Source: CAD feature listing. Evaluate the final solid. Frame: model axes, mm. Face numbers are marked on the shaded views. Give positions to 0.01 mm unless a question says otherwise; leave off trailing zeros. Loops run counter-clockwise (first coordinate to the right, second up) from the corner with the lowest first, then second, coordinate; pieces in that order, holes last. Notation, with made-up numbers: (29, 29.5) -> (87, 29.5) arc R24 cw to (87, 68.5) -> close; hole circle Ø7 at (43.5, 59). An arc over 180 degrees is marked (long way). Put each result on its own line as item: value.
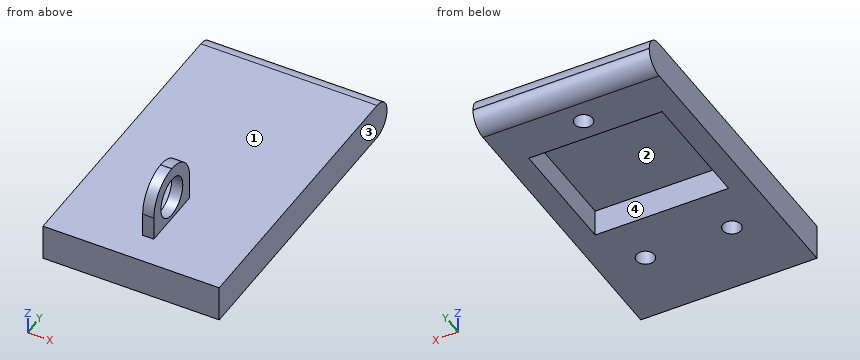
```python
from build123d import *

# Parameters (mm, degrees)
F0_W     = 3.1
F0_H     = 18.1
F1_DEPTH = 25.75
F0_W_2   = 48.9
F0_H_2   = 84.6
F2_DEPTH = 10.1
F3_R     = 5
F4_R     = 9
F5_R     = 5.499402
F6_DEPTH = 26.001
F7_R     = 2.5
F7_W     = 37
F7_H     = 33.5
F8_DEPTH = 7.5


with BuildPart() as f1:
    # F0 (on Top) → F1 (new body)
    with BuildSketch(Plane.XY):
        with Locations((23.972543, 18.115168)):
            Rectangle(F0_W, F0_H)
    extrude(amount=F1_DEPTH)

    # F0 (on Top) → F2 (join)
    with BuildSketch(Plane.XY):
        with Locations((23.972543, 42.723387)):
            Rectangle(F0_W_2, F0_H_2)
        with Locations((23.972543, 18.115168)):
            Rectangle(F0_W, F0_H, mode=Mode.SUBTRACT)
    extrude(amount=F2_DEPTH)

    # F3
    f3_edges = [f1.edges().sort_by_distance(p)[0] for p in [
        (23.972543, 85.023387, 10.1),
        (23.972543, 85.023387, 0),
    ]]
    fillet(f3_edges, radius=F3_R)

    # F4
    f4_edges = [f1.edges().sort_by_distance(p)[0] for p in [
        (23.972543, 9.065168, 25.75),
        (23.972543, 27.165168, 25.75),
    ]]
    fillet(f4_edges, radius=F4_R)

    # F5 (on face) → F6 (cut, through all)
    with BuildSketch(Plane.YZ.offset(25.522543)):
        with Locations((18.165168, 16.75)):
            Circle(F5_R)
    extrude(amount=-F6_DEPTH, mode=Mode.SUBTRACT)

    # F7 (on face) → F8 (cut)
    with BuildSketch(Plane.XY):
        with Locations((23.972543, 73.70657)):
            Circle(F7_R)
        with Locations((35.972543, 20.70657)):
            Circle(F7_R)
        with Locations((11.972543, 20.70657)):
            Circle(F7_R)
        with Locations((23.972543, 50.95657)):
            Rectangle(F7_W, F7_H)
    extrude(amount=F8_DEPTH, mode=Mode.SUBTRACT)


solid = f1.part
```
(1) Line query: probe 1 along X at (y, z) = (64, 1.5); probe 2 along X at (y, z) = (18.5, 5); probe 3 along X at (y, z) = (22, 11.5). Output: solid intervals per line, ascending. Write a range as from..to.
Calculated:
probe 1: x = -0.48..5.47, 42.47..48.42
probe 2: x = -0.48..10.8, 13.15..34.8, 37.15..48.42
probe 3: x = 22.42..25.52
(2) Draft query along X for the marked faces 1, 2, 3 and 4. Return one class per face: released by +X, released by -X, zero draft, split by the parting line, or undercut.
Calculated:
face 1: zero draft
face 2: undercut
face 3: released by +X
face 4: undercut
(3) Section A-A on x = 31. Return loops of the section in (y, z).
Calculated:
outline: (0.42, 0) -> (34.21, 0) -> (34.21, 7.5) -> (67.71, 7.5) -> (67.71, 0) -> (80.02, 0) arc R5 ccw to (85.02, 5) -> (85.02, 5.1) arc R5 ccw to (80.02, 10.1) -> (0.42, 10.1) -> close
(4) Section C-C on y = 38. Return loops of the section in (x, z), then the cut area to 3 significant figures.
Calculated:
outline: (-0.48, 0) -> (5.47, 0) -> (5.47, 7.5) -> (42.47, 7.5) -> (42.47, 0) -> (48.42, 0) -> (48.42, 10.1) -> (-0.48, 10.1) -> close
area: 216 mm²
(5) Section D-D on z = 3.5. Return loops of the section in (x, y), then the cut area to 3 significant figures.
Calculated:
outline: (-0.48, 0.42) -> (48.42, 0.42) -> (48.42, 84.79) -> (-0.48, 84.79) -> close; hole (5.47, 34.21) -> (42.47, 34.21) -> (42.47, 67.71) -> (5.47, 67.71) -> close; hole circle Ø5 at (11.97, 20.71); hole circle Ø5 at (23.97, 73.71); hole circle Ø5 at (35.97, 20.71)
area: 2,830 mm²
(6) First-contact query: P1, Ø8, axis at x = 11.97, y = 20.71, coming from the +Z side; P2, Ø10, axis at x = 24, y = 51, coming from the -Z side; P3, Ø0.9, axis at x = 24.5, z = 14, coming from the +Y side. Flat tips, straight axial feed; report the tip coordinate or a pass-through.
Calculated:
P1: stops at z = 10.1
P2: stops at z = 7.5
P3: stops at y = 27.17
(7) Section B-B on z = 21.25. Return loops of the section in (x, y), then the cut area to 3 significant figures.
Calculated:
outline: (22.42, 10.27) -> (25.52, 10.27) -> (25.52, 15) -> (22.42, 15) -> close; (22.42, 21.33) -> (25.52, 21.33) -> (25.52, 25.96) -> (22.42, 25.96) -> close
area: 29.0 mm²
